from build123d import *

# Parameters (mm, degrees)
SKETCH1_R           = 1.5
SKETCH1_R_2         = 2
BOSS_EXTRUDE1_DEPTH = 3.175
CUT_EXTRUDE1_DEPTH  = 4.175
CHAMFER1_SIZE       = 4


with BuildPart() as part:
    # Sketch1 → Boss-Extrude1 (new body)
    with BuildSketch(Plane.XY):
        Polygon((162, 162), (162, 92), (150, 80), (150, -80), (162, -92), (162, -162), (92, -162), (80, -150), (-80, -150), (-92, -162), (-162, -162), (-162, -92), (-150, -80), (-150, 80), (-162, 92), (-162, 162), (-92, 162), (-80, 150), (80, 150), (92, 162), align=None)
        with Locations((-157, 157)):
            Circle(SKETCH1_R, mode=Mode.SUBTRACT)
        with Locations((157, 157)):
            Circle(SKETCH1_R, mode=Mode.SUBTRACT)
        with Locations((157, -157)):
            Circle(SKETCH1_R, mode=Mode.SUBTRACT)
        with Locations((-157, -157)):
            Circle(SKETCH1_R, mode=Mode.SUBTRACT)
        with Locations((-91, 64)):
            Circle(SKETCH1_R_2, mode=Mode.SUBTRACT)
        with Locations((-91, 39)):
            Circle(SKETCH1_R_2, mode=Mode.SUBTRACT)
        with Locations((-59, 39)):
            Circle(SKETCH1_R_2, mode=Mode.SUBTRACT)
        with Locations((-59, 64)):
            Circle(SKETCH1_R_2, mode=Mode.SUBTRACT)
        with Locations((59, 39)):
            Circle(SKETCH1_R_2, mode=Mode.SUBTRACT)
        with Locations((59, 64)):
            Circle(SKETCH1_R_2, mode=Mode.SUBTRACT)
        with Locations((91, 39)):
            Circle(SKETCH1_R_2, mode=Mode.SUBTRACT)
        with Locations((91, 64)):
            Circle(SKETCH1_R_2, mode=Mode.SUBTRACT)
        with Locations((59, -64)):
            Circle(SKETCH1_R_2, mode=Mode.SUBTRACT)
        with Locations((59, -39)):
            Circle(SKETCH1_R_2, mode=Mode.SUBTRACT)
        with Locations((91, -39)):
            Circle(SKETCH1_R_2, mode=Mode.SUBTRACT)
        with Locations((91, -64)):
            Circle(SKETCH1_R_2, mode=Mode.SUBTRACT)
        with Locations((-91, -64)):
            Circle(SKETCH1_R_2, mode=Mode.SUBTRACT)
        with Locations((-59, -64)):
            Circle(SKETCH1_R_2, mode=Mode.SUBTRACT)
        with Locations((-59, -39)):
            Circle(SKETCH1_R_2, mode=Mode.SUBTRACT)
        with Locations((-91, -39)):
            Circle(SKETCH1_R_2, mode=Mode.SUBTRACT)
        with Locations((-33, -31)):
            Circle(SKETCH1_R_2, mode=Mode.SUBTRACT)
        Circle(SKETCH1_R_2, mode=Mode.SUBTRACT)
        with Locations((0, 49)):
            Circle(SKETCH1_R_2, mode=Mode.SUBTRACT)
        with Locations((0, -49)):
            Circle(SKETCH1_R_2, mode=Mode.SUBTRACT)
        with Locations((-147, 157)):
            Circle(SKETCH1_R, mode=Mode.SUBTRACT)
        with Locations((-157, 147)):
            Circle(SKETCH1_R, mode=Mode.SUBTRACT)
        with Locations((147, 157)):
            Circle(SKETCH1_R, mode=Mode.SUBTRACT)
        with Locations((157, 147)):
            Circle(SKETCH1_R, mode=Mode.SUBTRACT)
        with Locations((157, -147)):
            Circle(SKETCH1_R, mode=Mode.SUBTRACT)
        with Locations((147, -157)):
            Circle(SKETCH1_R, mode=Mode.SUBTRACT)
        with Locations((-147, -157)):
            Circle(SKETCH1_R, mode=Mode.SUBTRACT)
        with Locations((-157, -147)):
            Circle(SKETCH1_R, mode=Mode.SUBTRACT)
        with Locations((-142, 142)):
            Circle(SKETCH1_R, mode=Mode.SUBTRACT)
        with Locations((142, 142)):
            Circle(SKETCH1_R, mode=Mode.SUBTRACT)
        with Locations((142, -142)):
            Circle(SKETCH1_R, mode=Mode.SUBTRACT)
        with Locations((-142, -142)):
            Circle(SKETCH1_R, mode=Mode.SUBTRACT)
    extrude(amount=BOSS_EXTRUDE1_DEPTH)

    # Sketch2 → Cut-Extrude1 (cut, through all)
    with BuildSketch(Plane.XY.offset(3.175)):
        with BuildLine():
            Line((-156, 122), (-156, 107))
            ThreePointArc((-156, 107), (-154, 105), (-152, 107))
            Line((-152, 107), (-152, 122))
            ThreePointArc((-152, 122), (-154, 124), (-156, 122))
        make_face()
        with BuildLine():
            Line((-152, -107), (-152, -122))
            ThreePointArc((-152, -122), (-154, -124), (-156, -122))
            Line((-156, -122), (-156, -107))
            ThreePointArc((-156, -107), (-154, -105), (-152, -107))
        make_face()
    extrude(amount=-CUT_EXTRUDE1_DEPTH, mode=Mode.SUBTRACT)

    # Chamfer1
    chamfer1_edges = [part.edges().sort_by_distance(p)[0] for p in [
        (162, -162, 1.5875),
        (-162, -162, 1.5875),
        (-162, 162, 1.5875),
        (162, 162, 1.5875),
    ]]
    chamfer(chamfer1_edges, length=CHAMFER1_SIZE)


solid = part.part
CAD build for the part. Positions are in the model's coordinates, mm. A direction names the side the tool comes from. Give positions to 0.01 mm unless a question says otherwise; leave off trailing zeros. Loops run counter-clockwise (first coordinate to the right, second up) from the corner with the lowest first, then second, coordinate; pieces in that order, holes last. Notation, with made-up numbers: M -18,59 L -14,59 A18 cw -14,80 Z; hole C 34.5,82.5 d3. An arc over 180 degrees is marked long. Answer in a Markdown table with one row per item. Add a question column.
Item 1: Band-saw the part on B-B on y = -73.5. Give the cut face in (x, z) (3 decimals).
Item 2: Band-saw the part on A-A on z = 2.6. Give the number of separate pieces and of enclosed holes in the cut face, then the cut area to 3 significant figures.
Item 3: Probe probe 1 along Y at (x, z) = (-59, 1.7); probe 2 along X at (y, z) = (-142, 1.7). List the from-to ranges inside material, lowest first.
Item 4: Mould opens along Y. For faces 6 (the face through (2, 2, 0)), 7 (the face through (-86, 156, 2)), 8 (the face through (86, -156, 2)), 9 (the face through (156, -86, 2)) say: +Y half, -Y half, draft (parallel to the pull), parting line (faces both ways), or undercut.
Item 5: Drop flat-ended pins along their axis: P1, Ø3, axis at x = -91, y = -39, coming from the -Z side; P2, Ø1, axis at x = -18, z = 1, coming from the -Y side; P3, Ø2, axis at x = 19, y = -127.5, coming from the -Z side. Give the stop position or say it passes through.
Item 6: Tool access for faces 1 (the face through (-86, -156, 2)), 2 (the face through (156, 86, 2)), 3 (the face through (86, 156, 2)), 4 (the face through (2, 2, 3.175)), 5 (the face through (-156, -86, 2)): list every direction of +Z, -Z, +X, -X, +Y, -Y with a clear straight run to the whole face (end or side of a thin tool).
Reply:
| question | item | result |
|---|---|---|
| 1 | outline | M -150,0 L 150,0 L 150,3.175 L -150,3.175 Z |
| 2 | separate pieces | 1 |
| 2 | enclosed holes | 38 |
| 2 | area | 96,200 mm^2 |
| 3 | probe 1 | y = -150 to -66, -62 to -41, -37 to 37, 41 to 62, 66 to 150 |
| 3 | probe 2 | x = -162 to -143.5, -140.5 to 140.5, 143.5 to 162 |
| 4 | face 6 | draft |
| 4 | face 7 | +Y half |
| 4 | face 8 | -Y half |
| 4 | face 9 | undercut |
| 5 | P1 | passes through |
| 5 | P2 | stops at y = -150 |
| 5 | P3 | stops at z = 0 |
| 6 | face 1 | +Z, -Z, -Y |
| 6 | face 2 | +Z, -Z, +X |
| 6 | face 3 | +Z, -Z, +Y |
| 6 | face 4 | +Z, +X, -X, +Y, -Y |
| 6 | face 5 | +Z, -Z, -X |
